Autodesk Inventor part; units mm, degrees
ref_plane "YZ Plane" through (0, 0, 0) normal (1, 0, 0) x (0, 1, 0)
ref_plane "XZ Plane" through (0, 0, 0) normal (0, 1, 0) x (-1, 0, 0)
ref_plane "XY Plane" through (0, 0, 0) normal (0, 0, 1) x (1, 0, 0)
sketch "Sketch1" plane through (0, 0, 0) normal (0, 0, 1) x (1, 0, 0)
  line L0 (-46.5, -10) -> (46.5, -10)
  line L1 (46.5, -10) -> (46.5, 10)
  line L2 (46.5, 10) -> (-46.5, 10)
  line L3 (-46.5, 10) -> (-46.5, -10)
  line L4 (-46.5, -10) -> (46.5, 10) construction
  line L5 (46.5, -10) -> (-46.5, 10) construction
  line L6 (0, 0) -> (-57.93, 0) construction
  circle A0 centre (-36.5, 0) radius 2.75
  line L7 (0, 0) -> (0, 23.3519) construction
  circle A1 centre (36.5, 0) radius 2.75
  circle A2 centre (1.5, 0) radius 2.75
  dimension "d0" = 93
  dimension "d1" = 20
  dimension "d5" = 5.5
  dimension "d6" = 10
  dimension "d9" = 5.5
  dimension "d11" = 35
extrude "Extrusion1" add sketch "Sketch1" along normal blind 4 contours L3 L2 L1 L0 | A0 | A1 | A2
fillet "Fillet1" radius 10 4 edges at (-46.5, 10, 2) (-46.5, -10, 2) (46.5, 10, 2) (46.5, -10, 2)
extrude "Extrusion2" cut sketch "Sketch1" along normal through all contours A0 | A1 | A2
equation "\"d9\" = d5"
properties part number "encoder_link"
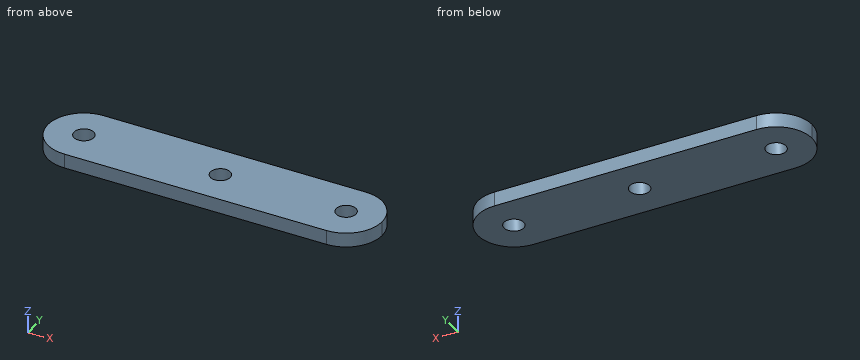
Geometry: final body of the model. Coordinates: model frame, mm. Give positions to 0.01 mm unless a question says otherwise; leave off trailing zeros. Order: outer loops, then holes, each group sorted by start corner. A loop starts at its lowest first (then second) coordinate and runs counter-clockwise, first axis right, second up. Notation, with made-up numbers: (5.5, 32) -> (26.5, 32) arc R32 cw to (26.5, 58) -> close; hole circle Ø1 at (24.5, 54.25). An arc over 180 degrees is marked (long way). Write each question's results on one line, items separated by ' | '.
1) Cut plane A-A (z = 1.2). Give the number of separate pieces and of enclosed holes in the cut face, and give its area (3 significant figures).
Geometry says:
separate pieces: 1 | enclosed holes: 3 | area: 1,700 mm²
2) Line query: line 1 along X through (y, z) = (0, 2.55); line 2 along Y through (x, z) = (-36.5, 2.5); line 3 along X through (y, z) = (-1, 3.65). Output: solid intervals per line, ascending.
Geometry says:
line 1: x = -46.5 to -39.25, -33.75 to -1.25, 4.25 to 33.75, 39.25 to 46.5 | line 2: y = -10 to -2.75, 2.75 to 10 | line 3: x = -46.45 to -39.06, -33.94 to -1.06, 4.06 to 33.94, 39.06 to 46.45
3) Cut plane C-C (y = -4.75). Output: boundary loops of the cut face in (x, z), and give its area (3 significant figures).
Geometry says:
outline: (-45.3, 0) -> (45.3, 0) -> (45.3, 4) -> (-45.3, 4) -> close | area: 362 mm²
4) Cut plane B-B (y = 5.5). Output: boundary loops of the cut face in (x, z), and give its area (3 significant figures).
Geometry says:
outline: (-44.85, 0) -> (44.85, 0) -> (44.85, 4) -> (-44.85, 4) -> close | area: 359 mm²
